```python
from build123d import *

# Parameters (mm, degrees)
SKETCH2_W                      = 127
SKETCH2_H                      = 76.2
BOSS_EXTRUDE2_DEPTH            = 76.2
FILLET1_R                      = 12.7
CHAMFER1_SIZE                  = 10
F_3_4_0_7500_DOWEL_HOLE1_D     = 19.05
F_3_4_0_7500_DOWEL_HOLE1_DEPTH = 76.2
F_3_4_0_7500_DOWEL_HOLE1_TIP   = 5.723197396
SKETCH9_W                      = 38.1
SKETCH9_H                      = 38.1
BOSS_EXTRUDE3_DEPTH            = 63.5
FILLET2_R                      = 3.302


# Read off the part's stored shape, not the designer's step: 1/4-20 Tapped Hole1
with BuildPart() as part:
    # Sketch2 → Boss-Extrude2 (new body)
    with BuildSketch(Plane(origin=(0, 0, 0), x_dir=(1, 0, 0), z_dir=(0, 1, 0))):
        Rectangle(SKETCH2_W, SKETCH2_H)
    extrude(amount=BOSS_EXTRUDE2_DEPTH)

    # Fillet1
    fillet1_edges = [part.edges().sort_by_distance(p)[0] for p in [
        (-63.5, 76.2, 0),
        (-63.5, 0, 0),
    ]]
    fillet(fillet1_edges, radius=FILLET1_R)

    # Chamfer1
    chamfer1_edges = [part.edges().sort_by_distance(p)[0] for p in [
        (-63.5, 38.1, 38.1),
        (-63.5, 38.1, -38.1),
        (6.35, 0, 38.1),
        (6.35, 76.2, 38.1),
        (-59.780256121, 72.480256121, 38.1),
        (-59.780256121, 3.719743879, 38.1),
        (-59.780256121, 72.480256121, -38.1),
        (-59.780256121, 3.719743879, -38.1),
        (6.35, 0, -38.1),
        (6.35, 76.2, -38.1),
    ]]
    chamfer(chamfer1_edges, length=CHAMFER1_SIZE)

    # 3/4 (0.7500) Dowel Hole1
    with Locations(Plane(origin=(63.5, 0, 0), x_dir=(0, 0, -1), z_dir=(1, 0, 0))):
        with Locations((0, 36.890636669)):
            Hole(F_3_4_0_7500_DOWEL_HOLE1_D / 2, depth=F_3_4_0_7500_DOWEL_HOLE1_DEPTH)
            with Locations((0, 0, -(F_3_4_0_7500_DOWEL_HOLE1_DEPTH + F_3_4_0_7500_DOWEL_HOLE1_TIP / 2))):  # 118° drill point
                Cone(0, F_3_4_0_7500_DOWEL_HOLE1_D / 2, F_3_4_0_7500_DOWEL_HOLE1_TIP, mode=Mode.SUBTRACT)

    # 1/4-20 Tapped Hole1 outline → 1/4-20 Tapped Hole1 (revolve, cut)
    with BuildSketch(Plane(origin=(9.290251981, 0, 0), x_dir=(1, 0, 0), z_dir=(0, 0, 1))):
        Polygon((2.145213652, 27.610479168), (0, 27.610479168), (0, 0), (2.5527, 0), (2.5527, 27.365636669), align=None)
    revolve(axis=Axis((9.290251981, 0, 0), (0, 1, 0)), mode=Mode.SUBTRACT)

    # 1_4-20 Tapped Hole1 2 outline → 1_4-20 Tapped Hole1 2 (revolve, cut)
    with BuildSketch(Plane(origin=(36.474004082, 0, 0), x_dir=(1, 0, 0), z_dir=(0, 0, 1))):
        Polygon((2.5527, 0), (2.5527, 27.365636669), (2.145213678, 27.610479152), (0, 27.610479152), (0, 0), align=None)
    revolve(axis=Axis((36.474004082, 0, 0), (0, 1, 0)), mode=Mode.SUBTRACT)

    # Sketch9 → Boss-Extrude3 (add)
    with BuildSketch(Plane(origin=(0, 76.2, 0), x_dir=(1, 0, 0), z_dir=(0, 1, 0))):
        Rectangle(SKETCH9_W, SKETCH9_H)
    extrude(amount=BOSS_EXTRUDE3_DEPTH)

    # Fillet2
    fillet2_edges = [part.edges().sort_by_distance(p)[0] for p in [
        (19.05, 76.2, 0),
        (-19.05, 76.2, 0),
        (19.05, 139.7, 0),
        (-19.05, 139.7, 0),
    ]]
    fillet(fillet2_edges, radius=FILLET2_R)


solid = part.part
```
For this review, take the finished solid that the model builds, in its own axes (mm). A direction names the side the tool comes from. Round coordinates to 2 decimals unless told otherwise and drop trailing zeros. Write each loop counter-clockwise with the first axis right and the second up, starting at its lowest first coordinate (ties: lowest second). Pieces come first, ordered by that corner, then holes. Notation, with made-up numbers: (66, 46) - (104, 46) arc R23 cw to (104, 74) - close; hole circle Ø5 at (43.5, 59). An arc over 180 degrees is marked (long way). Put each result on its own line as item: value.
Q1. Mouldability with a two-part tool opening along Z and no side actions: class faces 1 (the face through (11.725, 13.874, -0.767)), 2 (the face through (18.108, 138.707, -0.267)), 3 (the face through (-56.14, 7.25, 33.17)) as released by +Z, released by -Z, zero draft, split by the parting line, or undercut.
Solved:
face 1: undercut
face 2: zero draft
face 3: released by +Z
Q2. We need section C-C (x = 31). Give the boundary of the cut face in (y, z) (3 decimals), and give its area (3 significant figures).
Solved:
outline: (0, -28.1) - (10, -38.1) - (66.2, -38.1) - (76.2, -28.1) - (76.2, 28.1) - (66.2, 38.1) - (10, 38.1) - (0, 28.1) - close; hole circle Ø19.05 at (36.891, 0)
area: 5,320 mm2
Q3. Wall thickness on probe 1 along X at (y, z) = (20, 0); probe 2 along X at (y, z) = (6.75, 0); probe 3 along Z at (x, y) = (12, 97): over which ranges is each line inside the solid? List them lowest first.
Solved:
probe 1: x = -63.5 to 6.74, 11.84 to 33.92, 39.03 to 63.5
probe 2: x = -62.02 to 6.74, 11.84 to 33.92, 39.03 to 63.5
probe 3: z = -19.05 to 19.05
Q4. Insertion check: pin 1 Ø13.5 at (x, y) = (7.5, 99.5) entering from +Z; pin 2 Ø13.5 at (x, y) = (-5.5, 106) entering from -Z; pin 3 Ø3 at (x, y) = (-21, 116.5) entering from -Z; pin 4 Ø19 at (y, z) = (113.5, 5.5) entering from +X. Each pin has a flat end and moves straight along its axis. Give the tip position at first contact, or say it passes through.
Solved:
pin 1: stops at z = 19.05
pin 2: stops at z = -19.05
pin 3: passes through
pin 4: stops at x = 19.05
Q5. We need section A-A (x = -28.5). Give the boundary of the cut face in (y, z), and give its area (3 significant figures).
Solved:
outline: (0, -28.1) - (10, -38.1) - (66.2, -38.1) - (76.2, -28.1) - (76.2, 28.1) - (66.2, 38.1) - (10, 38.1) - (0, 28.1) - close
area: 5,610 mm2
Q6. Machinability: for faces 4 (the face through (19.05, 108, 0)), 5 (the face through (-19.05, 108, 0)), 6 (the face through (24.9, 27.6, -2.1)), which of the approach directions +Z, -Z, +X, -X, +Y, -Y give a long, thin tool a straight path to every point of the face, cutting with its end or side? Answer none if there is none.
Solved:
face 4: +Z, -Z, +X, +Y
face 5: +Z, -Z, -X, +Y
face 6: +X
Q7. We need section B-B (z = 13.5). Give the boundary of the cut face in (x, y), and give its area (3 significant figures).
Solved:
outline: (-63.5, 12.7) arc R12.7 ccw to (-50.8, 0) - (63.5, 0) - (63.5, 76.2) - (22.35, 76.2) arc R3.3 cw to (19.05, 79.5) - (19.05, 136.4) arc R3.3 ccw to (15.75, 139.7) - (-15.75, 139.7) arc R3.3 ccw to (-19.05, 136.4) - (-19.05, 79.5) arc R3.3 cw to (-22.35, 76.2) - (-50.8, 76.2) arc R12.7 ccw to (-63.5, 63.5) - close
area: 12,000 mm2
Q8. We need section D-D (y = 106). Give the boundary of the cut face in (x, z).
Solved:
outline: (-19.05, -19.05) - (19.05, -19.05) - (19.05, 19.05) - (-19.05, 19.05) - close
